Source: CAD feature listing. Evaluate the final solid. Frame: model axes, mm. A direction names the side the tool comes from. Round coordinates to 2 decimals unless told otherwise and drop trailing zeros. Loops run counter-clockwise (first coordinate to the right, second up) from the corner with the lowest first, then second, coordinate; pieces in that order, holes last. Notation, with made-up numbers: (39.5, 74) -> (45.5, 74) arc R16 ccw to (45.5, 85) -> close; hole circle Ø2 at (75, 16.25). An arc over 180 degrees is marked (long way). Put each result on its own line as item: value. Start each with the question number.
1. Draft query along Y for faces 1 (the cylindrical face through (-9.96, 1.43, 11.95)), 2 (the flat face through (0, -12.5, 7)), 3 (the flat face through (12.5, 0, 7)). Return one class per face: pulls with the +Y half, pulls with the -Y half, needs draft (parallel to the pull), parting line crosses it, or undercut.
2. Cut plane D-D (y = 0). Return the cut outline in (x, z), then the cut area to 3 significant figures.
3. Cut plane B-B (y = 6.7). Return the cut outline in (x, z), then the cut area to 3 significant figures.
4. Material intervals for L1, parallel to X at y = -3, z = 7.25; L2, parallel to Y at x = 10.7, z = 3.5; L3, parallel to X at y = -6.7, z = 9, sorted ascending.
5. Contact query for flat-ended pins moving along their axis: pin 1 (1.5 mm diameter, centred on x = -6.5, y = -8, fed in from +Z); pin 2 (2.5 mm diameter, centred on x = -6.7, y = -6.7, fed in from +Z). Output: stop coordinate, or through.
6. Set-up query: faces 4 (the cylindrical face through (-9.965, -0.575, 2.114)), 5 (the flat face through (7.5, 0, 7)). Return all of +Z, -Z, +X, -X, +Y, -Y with unobstructed straight access to the full face (end or side cutting, diameter ignored); none if empty.
7. Cut plane A-A (z = 11.5). Return the cut outline in (x, y).
```python
from build123d import *

# Parameters (mm, degrees)
SKETCH_1_W          = 25
SKETCH_1_H          = 25
SKETCH_1_W_2        = 15
SKETCH_1_H_2        = 15
EXTRUDE_1_DEPTH     = 15
SKETCH_2_R          = 1.5
CUT_EXTRUDE_1_DEPTH = 24.184046239
SKETCH_3_R          = 1.5
CUT_EXTRUDE_2_DEPTH = 32.721443851


with BuildPart() as part:
    # 草图1 → 凸台-拉伸1 (new body)
    with BuildSketch(Plane.XY):
        Rectangle(SKETCH_1_W, SKETCH_1_H)
        Rectangle(SKETCH_1_W_2, SKETCH_1_H_2, mode=Mode.SUBTRACT)
    extrude(amount=EXTRUDE_1_DEPTH)

    # 草图2 → 切除-拉伸1 (cut, through all)
    with BuildSketch(Plane.XY.offset(15)):
        with Locations((6.7, 6.7)):
            Circle(SKETCH_2_R)
        with Locations((6.7, -6.7)):
            Circle(SKETCH_2_R)
        with Locations((-6.7, -6.7)):
            Circle(SKETCH_2_R)
        with Locations((-6.7, 6.7)):
            Circle(SKETCH_2_R)
    extrude(amount=-CUT_EXTRUDE_1_DEPTH, mode=Mode.SUBTRACT)

    # 草图3 → 切除-拉伸2 (cut, through all)
    with BuildSketch(Plane(origin=(12.5, 0, 0), x_dir=(0, 0, -1), z_dir=(1, 0, 0))):
        with Locations(Location((-11.5, 0, 0), (0, 0, 90))):
            Circle(SKETCH_3_R)
        with Locations((-3.5, 0)):
            Circle(SKETCH_3_R)
    extrude(amount=-CUT_EXTRUDE_2_DEPTH, mode=Mode.SUBTRACT)


solid = part.part
```
Solution:
1. face 1: undercut
1. face 2: pulls with the -Y half
1. face 3: needs draft
2. outline: (-12.5, 0) -> (-7.5, 0) -> (-7.5, 2) -> (-12.5, 2) -> close; (-12.5, 5) -> (-7.5, 5) -> (-7.5, 10) -> (-12.5, 10) -> close; (-12.5, 13) -> (-7.5, 13) -> (-7.5, 15) -> (-12.5, 15) -> close; (7.5, 0) -> (12.5, 0) -> (12.5, 2) -> (7.5, 2) -> close; (7.5, 5) -> (12.5, 5) -> (12.5, 10) -> (7.5, 10) -> close; (7.5, 13) -> (12.5, 13) -> (12.5, 15) -> (7.5, 15) -> close
2. area: 90.0 mm^2
3. outline: (-12.5, 0) -> (-8.2, 0) -> (-8.2, 15) -> (-12.5, 15) -> close; (8.2, 0) -> (12.5, 0) -> (12.5, 15) -> (8.2, 15) -> close
3. area: 129 mm^2
4. L1: x = -12.5 to -7.5, 7.5 to 12.5
4. L2: y = -12.5 to -1.5, 1.5 to 12.5
4. L3: x = -12.5 to -8.2, 8.2 to 12.5
5. pin 1: stops at z = 15
5. pin 2: passes through
6. face 4: +X, -X
6. face 5: +Z, -Z
7. outline: (-12.5, -12.5) -> (12.5, -12.5) -> (12.5, -1.5) -> (7.5, -1.5) -> (7.5, -5.43) arc R1.5 cw (long way) to (5.43, -7.5) -> (-5.43, -7.5) arc R1.5 cw (long way) to (-7.5, -5.43) -> (-7.5, -1.5) -> (-12.5, -1.5) -> close; (-12.5, 1.5) -> (-7.5, 1.5) -> (-7.5, 5.43) arc R1.5 cw (long way) to (-5.43, 7.5) -> (5.43, 7.5) arc R1.5 cw (long way) to (7.5, 5.43) -> (7.5, 1.5) -> (12.5, 1.5) -> (12.5, 12.5) -> (-12.5, 12.5) -> close
